```python
from build123d import *

# Parameters (mm, degrees)
SKETCH_1_R               = 2
EXTRUDE_1_DEPTH          = 16
EXTRUDE_2_DEPTH          = 3.175
SKETCH_4_R               = 1.65
CUT_EXTRUDE_6_DEPTH      = 2.5
SKETCH_5_W               = 10.65
SKETCH_5_H               = 0.5
CUT_EXTRUDE_8_DEPTH      = 9.5
FILLET_3_R               = 0.6
SKETCH_7_R               = 3.175
EXTRUDE_3_DEPTH          = 1.4
FILLET_5_R               = 0.3
CUT_EXTRUDE_9_DEPTH      = 1
CUT_EXTRUDE_9_DEPTH_BACK = 25.5
CUT_EXTRUDE_10_DEPTH     = 9.5
CUT_EXTRUDE_11_DEPTH     = 0.3
FILLET_6_R               = 1
CUT_EXTRUDE_12_DEPTH     = 0.5


with BuildPart() as part:
    # 草图1 → 凸台-拉伸1 (new body)
    with BuildSketch(Plane(origin=(0, 0, 0), x_dir=(1, 0, 0), z_dir=(0, 1, 0))):
        Circle(SKETCH_1_R)
    extrude(amount=EXTRUDE_1_DEPTH)

    # 草图2 → 凸台-拉伸2 (add)
    with BuildSketch(Plane.XY):
        with BuildLine():
            Line((3.175, 16), (0.486277818, 22.110914255))
            ThreePointArc((0.486277818, 22.110914255), (-6.524899776, 22.6859029), (-3.175, 16.5))
            Line((-3.175, 16.5), (-3.175, 16))
            Line((-3.175, 16), (3.175, 16))
        make_face()
    extrude(amount=EXTRUDE_2_DEPTH)

    # 草图4 → 切除-拉伸6 (cut)
    with BuildSketch(Plane(origin=(0, 0, 0), x_dir=(-1, 0, 0), z_dir=(0, 0, -1))):
        with Locations((3.175, 20.5)):
            Circle(SKETCH_4_R)
    extrude(amount=-CUT_EXTRUDE_6_DEPTH, mode=Mode.SUBTRACT)

    # 草图5 → 切除-拉伸8 (cut, through all)
    with BuildSketch(Plane(origin=(0, 16, 0), x_dir=(1, 0, 0), z_dir=(0, 1, 0))):
        with Locations((-2.15, -0.25)):
            Rectangle(SKETCH_5_W, SKETCH_5_H)
    extrude(amount=CUT_EXTRUDE_8_DEPTH, mode=Mode.SUBTRACT)

    # 圆角3
    fillet_3_edges = [part.edges().sort_by_distance(p)[0] for p in [
        (-2, 0, 0),
    ]]
    fillet(fillet_3_edges, radius=FILLET_3_R)

    # 草图7 → 凸台-拉伸3 (add)
    with BuildSketch(Plane(origin=(0, 16, 0), x_dir=(1, 0, 0), z_dir=(0, 1, 0))):
        Circle(SKETCH_7_R)
    extrude(amount=-EXTRUDE_3_DEPTH)

    # 圆角5
    fillet_5_edges = [part.edges().sort_by_distance(p)[0] for p in [
        (-1.525, 20.5, 0.5),
    ]]
    fillet(fillet_5_edges, radius=FILLET_5_R)

    # 草图10 → 切除-拉伸9 (cut, two sides)
    with BuildSketch(Plane.XZ) as cut_extrude_9_sk:
        with BuildLine():
            Line((-1.307669683, 0.5), (1.307669683, 0.5))
            ThreePointArc((1.307669683, 0.5), (0, -1.4), (-1.307669683, 0.5))
        make_face()
    extrude(amount=CUT_EXTRUDE_9_DEPTH, mode=Mode.SUBTRACT)
    extrude(cut_extrude_9_sk.sketch, amount=-CUT_EXTRUDE_9_DEPTH_BACK, mode=Mode.SUBTRACT)

    # 草图11 → 切除-拉伸10 (cut, through all)
    with BuildSketch(Plane.XZ.offset(-16)):
        with BuildLine():
            Line((3.175, 3.175), (0, 3.175))
            ThreePointArc((0, 3.175), (2.060718928, 2.415380405), (3.135382752, 0.5))
            Line((3.135382752, 0.5), (4.008589629, 0.5))
            Line((4.008589629, 0.5), (3.175, 3.175))
        make_face()
    extrude(amount=-CUT_EXTRUDE_10_DEPTH, mode=Mode.SUBTRACT)

    # 草图12 → 切除-拉伸11 (cut)
    with BuildSketch(Plane(origin=(0, 16, 0), x_dir=(1, 0, 0), z_dir=(0, 1, 0))):
        with BuildLine():
            Line((-3.135382752, -0.5), (3.135382752, -0.5))
            ThreePointArc((3.135382752, -0.5), (0, 3.175), (-3.135382752, -0.5))
        make_face()
    extrude(amount=-CUT_EXTRUDE_11_DEPTH, mode=Mode.SUBTRACT)

    # 圆角6
    fillet_6_edges = [part.edges().sort_by_distance(p)[0] for p in [
        (0, 15.7, -1.4),
    ]]
    fillet(fillet_6_edges, radius=FILLET_6_R)

    # 草图13 → 切除-拉伸12 (cut)
    with BuildSketch(Plane.XZ.offset(-16)):
        with BuildLine():
            Line((-3.135382752, 0.5), (-3.175, 0.5))
            Line((-3.175, 0.5), (-3.175, 3.175))
            Line((-3.175, 3.175), (0, 3.175))
            ThreePointArc((0, 3.175), (-2.060718928, 2.415380405), (-3.135382752, 0.5))
        make_face()
    extrude(amount=-CUT_EXTRUDE_12_DEPTH, mode=Mode.SUBTRACT)


solid = part.part
```
Geometry check sheet. Reference: the model listing, model coordinates, mm. A direction names the side the tool comes from. Give positions to 0.01 mm unless a question says otherwise; leave off trailing zeros. Order: outer loops, then holes, each group sorted by start corner. A loop starts at its lowest first (then second) coordinate and runs counter-clockwise, first axis right, second up. Notation, with made-up numbers: (-14.75, 49) - (12.25, 49) arc R8 ccw to (12.25, 61) - close; hole circle Ø11 at (-16.75, 22.25). An arc over 180 degrees is marked (long way). Answer in a Markdown table with one row per item. Add a question column.
Q1. Material ranges on probe 1 along Y at (x, z) = (-3.25, 1); probe 2 along X at (y, z) = (5.25, 0); probe 3 along Z at (x, y) = (0, 4.25), recorded low to high. Write a range as from..to.
Q2. Cross-section at C-C, the plane y = 6.25. Enter the section's corners in (x, z).
Q3. Cross-section at B-B, the plane x = 2.75. Enter the section's corners in (y, z), then the cut area to 3 significant figures.
Q4. Cross-section at A-A, the plane z = 2.25. Enter the section's corners in (x, y) (3 decimals), then the cut area to 3 significant figures.
Q5. Tool access check on faces 5 (the flat face through (0, 15.7, -3)), 6 (the cylindrical face through (-2.96, 22.136, 1.638)), 7 (the flat face through (1, 14.6, 2)). Record the directions out of +Z, -Z, +X, -X, +Y, -Y that give a thin tool (end or side, any length) a straight path to the whole face; none if there is none.
Q6. Mould release check, pull along Z, two halves, no side actions. Record for faces 1 (the cylindrical face through (0, 7.2, -1.4)), 2 (the flat face through (0, 0, 1)), 3 (the flat face through (-4, 21, 3.175)), 4 (the cylindrical face through (0, 8, 2)): pulls with the +Z half, pulls with the -Z half, needs draft (parallel to the pull), parting line crosses it, or undercut.
Q7. Gauge pin test, flat ends, axial feed: pin 1 (1 mm diameter, centred on x = 2, z = 0.5, fed in from +Y); pin 2 (1.8 mm diameter, centred on x = 1.5, z = -1, fed in from +Y); pin 3 (1.6 mm diameter, centred on x = -3.5, y = 20, fed in from -Z). Record the tip position at first contact, or that the pin passes through.
Check values:
| question | item | result |
|---|---|---|
| 1 | probe 1 | y = 16.5..18.85, 22.15..24.5 |
| 1 | probe 2 | x = -2..-1.4, 1.4..2 |
| 1 | probe 3 | z = -2..-1.4, 0.5..2 |
| 2 | outline | circle Ø4 at (0, 0); hole (-1.31, 0.5) arc R1.4 ccw (long way) to (1.31, 0.5) - close |
| 3 | outline | (14.6, -1.59) - (15.7, -1.59) - (15.7, 0.5) - (16.97, 0.5) - (16.97, 1.59) - (14.6, 1.59) - close |
| 3 | area | 4.87 mm^2 |
| 4 | outline | (-3.175, 16.5) - (-2.24, 16.5) - (-2.24, 14.6) - (2.24, 14.6) - (2.24, 18.125) - (0.486, 22.111) arc R4 ccw (long way) to start; hole circle Ø3.3 at (-3.175, 20.5) |
| 4 | area | 58.3 mm^2 |
| 5 | face 5 | -Z, +X, -X, +Y |
| 5 | face 6 | -Z |
| 5 | face 7 | -Y |
| 6 | face 1 | undercut |
| 6 | face 2 | needs draft |
| 6 | face 3 | pulls with the +Z half |
| 6 | face 4 | parting line crosses it |
| 7 | pin 1 | stops at y = 19.81 |
| 7 | pin 2 | stops at y = 15.7 |
| 7 | pin 3 | stops at z = 2.5 |
